Geometry: final body of the model. Coordinates: model frame, mm. A direction names the side the tool comes from. Give positions to 0.01 mm unless a question says otherwise; leave off trailing zeros. Order: outer loops, then holes, each group sorted by start corner. A loop starts at its lowest first (then second) coordinate and runs counter-clockwise, first axis right, second up. Notation, with made-up numbers: (-6, 85) - (33, 85) arc R21 ccw to (33, 119) - close; hole circle Ø9 at (73, -13). An arc over 180 degrees is marked (long way). One line per question, with ' | ' between items. Start each with the question number.
from build123d import *

# Parameters (mm, degrees)
SKETCH_2_R          = 11.5
SKETCH_2_R_2        = 1.7
CUT_EXTRUDE_1_DEPTH = 65.2579178


with BuildPart() as part:
    # 草图1 → 旋转1 (revolve)
    with BuildSketch(Plane.XY, mode=Mode.PRIVATE) as revolve_1_sk:
        Polygon((39.8, 31), (39.8, 0), (0, 0), (0, 3), (33.8, 3), (33.8, 31), align=None)
    revolve(revolve_1_sk.sketch.rotate(Axis((0, 0, 0), (0, 1, 0)), 90), axis=Axis((0, 0, 0), (0, 1, 0)))

    # 草图2 → 切除-拉伸1 (cut, through all)
    with BuildSketch(Plane.XZ):
        with Locations(Location((0, 0, 0), (0, 0, 270))):
            Circle(SKETCH_2_R)
        with Locations(Location((0, 20, 0), (0, 0, 270))):
            Circle(SKETCH_2_R_2)
        with Locations(Location((17.320508076, -10, 0), (0, 0, 270))):
            Circle(SKETCH_2_R_2)
        with Locations(Location((-17.320508076, -10, 0), (0, 0, 270))):
            Circle(SKETCH_2_R_2)
    extrude(amount=-CUT_EXTRUDE_1_DEPTH, mode=Mode.SUBTRACT)


solid = part.part
(1) Access query for faces 1 (the cylindrical face through (19.006, 1.479, -9.779)), 2 (the flat face through (0, 3, 15)). Directions: +Z, -Z, +X, -X, +Y, -Y. A direction counts if a zero-diameter tool reaches every point of the face in a straight line with its end or side. Return the directions, or none.
(2) Cut plane A-A, the plane z = 0. Return the cut outline in (x, y).
(3) Cut plane B-B, the plane x = 0. Return the cut outline in (y, z), plus the area to 3 significant figures.
(4) Cut plane D-D, the plane z = 20. Return the cut outline in (x, y).
(5) Contact query for flat-ended pins moving along their axis: P1, Ø10, axis at x = -8.5, z = -16.5, coming from the +Y side; P2, Ø8, axis at x = -4.5, y = 21.5, coming from the +Z side; P3, Ø2, axis at x = -15, y = 28, coming from the +Z side; P4, Ø1, axis at x = 25, z = -31.5, coming from the -Y side. Output: stop coordinate, or through.
(6) Material intervals for line 1 along X through (y, z) = (12.5, 0); line 2 along X through (y, z) = (1, -10); line 3 along Y through (x, z) = (21, 3.5), sorted ascending. Write a range as from..to.
(7) Cut plane C-C, the plane y = 5. Return the cut outline in (x, z).
(8) Pull-direction query (X, two-part tool) for faces 3 (the flat face through (8.3, 0, -8.3)), 4 (the cylindrical face through (-0.65, 1.48, 18.43)), 5 (the cylindrical face through (24.22, 15.28, 31.58)), 6 (the cylindrical face through (-18.98, 1.48, -9.63)); classes: +X half, -X half, draft (parallel to the pull), parting line (faces both ways), or undercut.
Results are:
1) face 1: +Y, -Y | face 2: +Y
2) outline: (-39.8, 0) - (-11.5, 0) - (-11.5, 3) - (-33.8, 3) - (-33.8, 31) - (-39.8, 31) - close; (11.5, 0) - (39.8, 0) - (39.8, 31) - (33.8, 31) - (33.8, 3) - (11.5, 3) - close
3) outline: (0, -39.8) - (31, -39.8) - (31, -33.8) - (3, -33.8) - (3, -11.5) - (0, -11.5) - close; (0, 11.5) - (3, 11.5) - (3, 18.3) - (0, 18.3) - close; (0, 21.7) - (3, 21.7) - (3, 33.8) - (31, 33.8) - (31, 39.8) - (0, 39.8) - close | area: 496 mm2
4) outline: (-34.41, 0) - (-1.7, 0) - (-1.7, 3) - (-27.25, 3) - (-27.25, 31) - (-34.41, 31) - close; (1.7, 0) - (34.41, 0) - (34.41, 31) - (27.25, 31) - (27.25, 3) - (1.7, 3) - close
5) P1: y = 3 | P2: z = 39.8 | P3: z = 37.26 | P4: y = 0
6) line 1: -39.8..-33.8, 33.8..39.8 | line 2: -38.52..-19.02, -15.62..-5.68, 5.68..15.62, 19.02..38.52 | line 3: 0..3
7) outline: circle Ø79.6 at (0, 0); hole circle Ø67.6 at (0, 0)
8) face 3: draft | face 4: undercut | face 5: parting line | face 6: undercut
